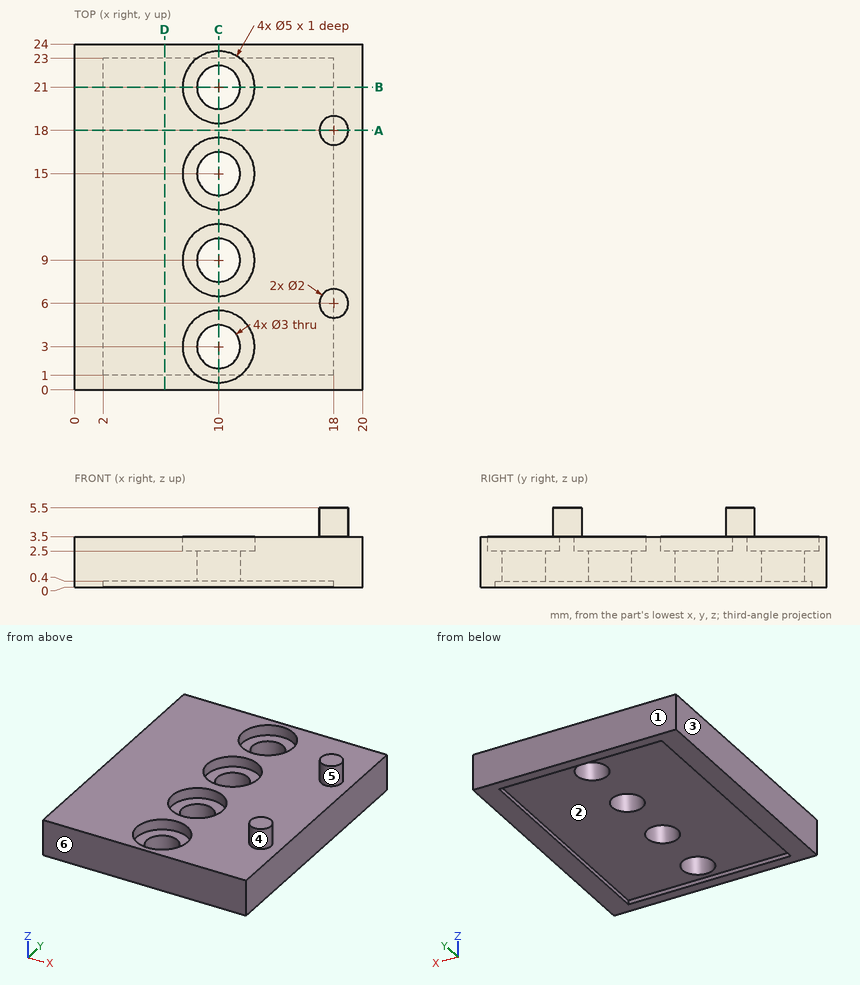
For this review, use the dimensioned drawing (mm, ordinates from the lowest corner) and the shaded views. A direction names the side the tool comes from. Round coordinates to 2 decimals unless told otherwise and drop trailing zeros. Order: outer loops, then holes, each group sorted by start corner. A loop starts at its lowest first (then second) coordinate and runs counter-clockwise, first axis right, second up. Notation, with made-up numbers: M 36.25,54 L 45.25,54 A33 cw 45.25,91 Z; hole C 7.5,1 d5. An arc over 180 degrees is marked long. Use a Markdown table: item, result. Add a question column.
Item 1: Add section B-B, the plane y = 21. Give the boundary of the cut face in (x, z).
Item 2: To check wall thickness, follow line 1 along Y through (x, z) = (10, 2); line 2 along Y through (x, z) = (10, 3.25); line 3 along X through (y, z) = (9, 1.85). State the ranges of each line that lie inside material, in increasing order.
Item 3: Mouldability with a two-part tool opening along Y and no side actions: class the marked faces 1, 2, 3 and 4 as released by +Y, released by -Y, zero draft, split by the parting line, or undercut.
Item 4: Add section C-C, the plane x = 10. State how many separate pieces and enclosed holes the cut face has, then the cut area to 3 significant figures.
Item 5: Add section A-A, the plane y = 18. Give the boundary of the cut face in (x, z), then the cut area to 3 significant figures.
Item 6: Add section D-D, the plane x = 6.25. Give the boundary of the cut face in (y, z).
Item 7: Tool access review of the marked faces 5 and 6: name each direction out of +Z, -Z, +X, -X, +Y, -Y from which nothing blocks a thin tool from reaching the whole face with its end or side.
Item 8: Insertion check: pin 1 (6.5 mm diameter, centred on x = 10, y = 21, fed in from +Z); pin 2 (5 mm diameter, centred on x = 14.5, y = 12, fed in from -Z); pin 3 (1.5 mm diameter, centred on y = 21, z = 1, fed in from -X); pin 4 (2.5 mm diameter, centred on x = 10.5, y = 3.5, fed in from +Z). Each pin has a flat end and moves straight along its axis. Give the tip position at first contact, or say it passes through.
Geometry results:
| question | item | result |
|---|---|---|
| 1 | outline | M 0,0 L 2,0 L 2,0.4 L 8.5,0.4 L 8.5,2.5 L 7.5,2.5 L 7.5,3.5 L 0,3.5 Z; M 11.5,0.4 L 18,0.4 L 18,0 L 20,0 L 20,3.5 L 12.5,3.5 L 12.5,2.5 L 11.5,2.5 Z |
| 2 | line 1 | y = 0 to 1.5, 4.5 to 7.5, 10.5 to 13.5, 16.5 to 19.5, 22.5 to 24 |
| 2 | line 2 | y = 0 to 0.5, 5.5 to 6.5, 11.5 to 12.5, 17.5 to 18.5, 23.5 to 24 |
| 2 | line 3 | x = 0 to 8.5, 11.5 to 20 |
| 3 | face 1 | released by +Y |
| 3 | face 2 | undercut |
| 3 | face 3 | zero draft |
| 3 | face 4 | undercut |
| 4 | separate pieces | 5 |
| 4 | enclosed holes | 0 |
| 4 | area | 30.0 mm² |
| 5 | outline | M 0,0 L 2,0 L 2,0.4 L 18,0.4 L 18,0 L 20,0 L 20,3.5 L 19,3.5 L 19,5.5 L 17,5.5 L 17,3.5 L 0,3.5 Z |
| 5 | area | 67.6 mm² |
| 6 | outline | M 0,0 L 1,0 L 1,0.4 L 23,0.4 L 23,0 L 24,0 L 24,3.5 L 0,3.5 Z |
| 7 | face 5 | +Z |
| 7 | face 6 | +Z, -Z, +X, -X, -Y |
| 8 | pin 1 | stops at z = 3.5 |
| 8 | pin 2 | stops at z = 0.4 |
| 8 | pin 3 | stops at x = 0 |
| 8 | pin 4 | stops at z = 2.5 |
